Source: CAD feature listing. Evaluate the final solid. Frame: model axes, mm. Round coordinates to 2 decimals unless told otherwise and drop trailing zeros. Loops run counter-clockwise (first coordinate to the right, second up) from the corner with the lowest first, then second, coordinate; pieces in that order, holes last. Notation, with made-up numbers: M -23,-26 L -5,-26 A30 ccw -5,0 Z; hole C 32,69 d5. An arc over 180 degrees is marked long. One line per item, written item: value.
Autodesk Inventor part; units mm, degrees
ref_plane "YZ Plane" through (0, 0, 0) normal (1, 0, 0) x (0, 1, 0)
ref_plane "XZ Plane" through (0, 0, 0) normal (0, 1, 0) x (-1, 0, 0)
ref_plane "XY Plane" through (0, 0, 0) normal (0, 0, 1) x (1, 0, 0)
sketch "Skizze1" plane through (0, 0, 0) normal (0, 0, 1) x (1, 0, 0)
  line L0 (0, -5) -> (0, 5) construction
  line L1 (6.3, -5) -> (6.3, 5)
  line L2 (-6.3, 5) -> (-6.3, -5)
  arc A0 (-6.3, -5) -> (6.3, -5) centre (0, -5) ccw
  arc A1 (6.3, 5) -> (-6.3, 5) centre (0, 5) ccw
  point P0 (0, 0)
  dimension "d0" = 12.6
  dimension "d1" = 10
extrude "Extrusion1" add sketch "Skizze1" along normal blind 5
sketch "Skizze2" plane through (0, 0, 5) normal (0, 0, 1) x (1, 0, 0)
  arc A0 (6.3, 5) -> (-6.3, 5) centre (0, 5) ccw
  arc A1 (-6.3, -5) -> (6.3, -5) centre (0, -5) ccw
  line L0 (0, 5.5) -> (0, -4) construction
  point P0 (0, 0)
  dimension "d11" = 9.5
  dimension "d13" = 1
hole "Bohrung1" at (0, 5.5, 5) at (0, -4, 5) direction (0, 0, -1) diameter 3.3 end through all countersink diameter 7 countersink angle 90
properties part number "Dribbler Slider" material "Gummi, Silikon"
1. Ray query, line 1 (Y direction, x = 0, z = 1.8); line 2 (Y direction, x = 1, z = 4.2); line 3 (X direction, y = -4, z = 2.4). Return the intervals inside material, ascending. Write a range as [from, to].
Report:
line 1: y = [-11.3, -5.65], [-2.35, 3.85], [7.15, 11.3]
line 2: y = [-11.22, -6.51], [-1.49, 2.99], [8.01, 11.22]
line 3: x = [-6.3, -1.65], [1.65, 6.3]
2. Section query A-A (x = 0). Return the cut outline in (y, z).
Report:
outline: M -11.3,0 L -5.65,0 L -5.65,3.15 L -7.5,5 L -11.3,5 Z; M -2.35,0 L 3.85,0 L 3.85,3.15 L 2,5 L -0.5,5 L -2.35,3.15 Z; M 7.15,0 L 11.3,0 L 11.3,5 L 9,5 L 7.15,3.15 Z
3. Section query D-D (y = 5.5). Return the cut outline in (x, z), and give its area (3 significant figures).
Report:
outline: M -6.28,0 L -1.65,0 L -1.65,3.15 L -3.5,5 L -6.28,5 Z; M 1.65,0 L 6.28,0 L 6.28,5 L 3.5,5 L 1.65,3.15 Z
area: 42.9 mm2
4. Section query B-B (z = 3.6). Return the cut outline in (x, y).
Report:
outline: M -6.3,-5 A6.3 ccw 6.3,-5 L 6.3,5 A6.3 ccw -6.3,5 Z; hole C 0,-4 d4.2; hole C 0,5.5 d4.2
5. Section query C-C (y = -4). Return the cut outline in (x, z).
Report:
outline: M -6.3,0 L -1.65,0 L -1.65,3.15 L -3.5,5 L -6.3,5 Z; M 1.65,0 L 6.3,0 L 6.3,5 L 3.5,5 L 1.65,3.15 Z
6. Pull-direction query (Y, two-part tool) for faces 1 (the face through (0, 0, 5)), 2 (the face through (0.1, -11.3, 2.5)), 3 (the face through (-1.724, 5.883, 3.266)), 4 (the face through (-1.074, -2.599, 3.266)); classes: released by +Y, released by -Y, zero draft, split by the parting line, or undercut.
Report:
face 1: zero draft
face 2: released by -Y
face 3: undercut
face 4: undercut
7. Pin query (flat end, axial travel): pin 1 (2 mm diameter, centred on x = 0, y = 5.5, fed in from -Z); pin 2 (4.5 mm diameter, centred on x = 0, y = -4, fed in from +Z); pin 3 (3 mm diameter, centred on x = 2, z = 2, fed in from -Y); pin 4 (2 mm diameter, centred on x = -2, z = 1.5, fed in from +Y). Return the tip coordinate at first contact, or that it passes through.
Report:
pin 1: passes through
pin 2: stops at z = 3.75
pin 3: stops at y = -11.28
pin 4: stops at y = 11.22
